The drawing under review shows one solid part. Ordinate dimensions are in mm from its lowest x, y, z. Round coordinates to 2 decimals unless told otherwise and drop trailing zeros. Write each loop counter-clockwise with the first axis right and the second up, starting at its lowest first coordinate (ties: lowest second). Pieces come first, ordered by that corner, then holes. Notation, with made-up numbers: (6, -37) -> (24, -37) arc R26 cw to (24, -14) -> close; hole circle Ø2 at (53.5, -20). An arc over 180 degrees is marked (long way). Use CSV: the item, a comma, the result in double quotes. Start each with the question number.
1) Mouldability with a two-part tool opening along Z and no side actions: class the marked faces 1, 2 and 3 as released by +Z, released by -Z, zero draft, split by the parting line, or undercut.
2) Wall thickness on probe 1 along Z at (x, y) = (1.5, 0.8); probe 2 along Y at (x, z) = (1, 3); probe 3 along Z at (x, y) = (1.05, 0.25): over which ranges is each line inside the solid? List them lowest first. Write a range as [from, to].
3) Take a section at C-C, the plane z = 12.75. Give the boundary of the cut face in (x, y).
4) Take a section at A-A, the plane x = 1. Give the boundary of the cut face in (y, z).
5) For pin 1 Ø1 at (x, z) = (1.5, 14.5) entering from +Y, flat-tipped, find the tip position at first contact; note if it passes through.
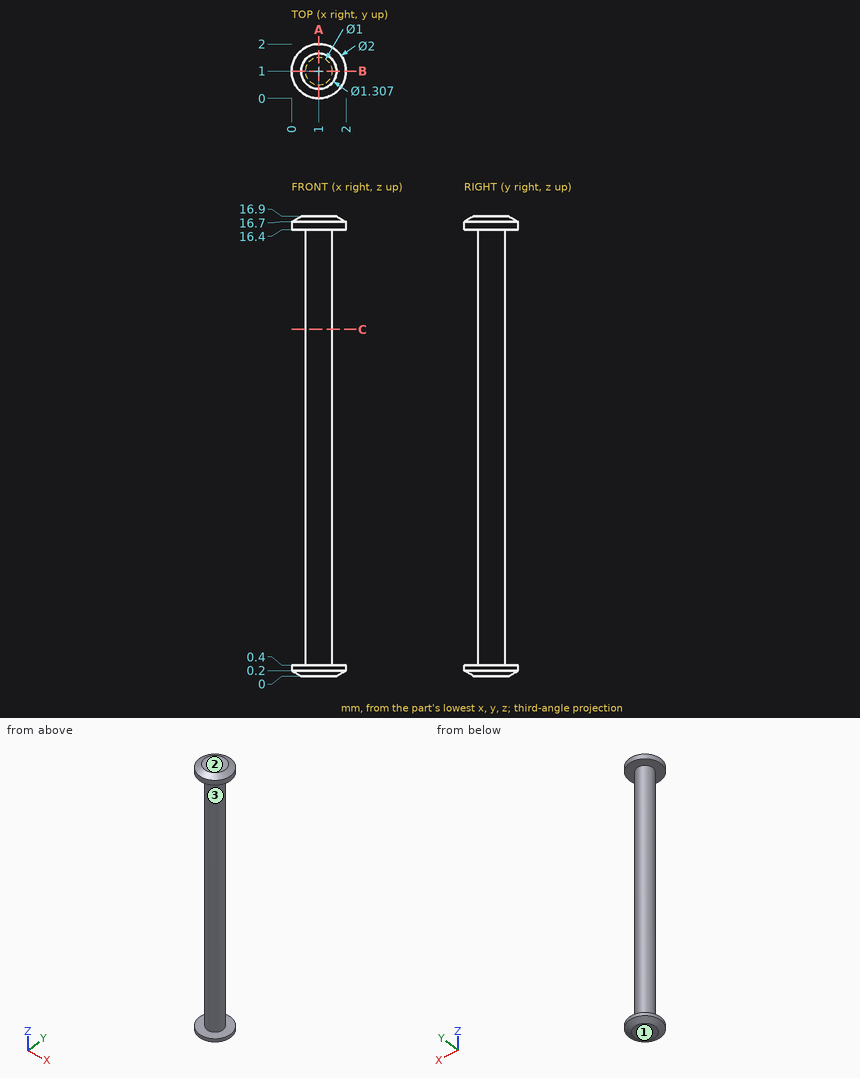
Values found:
1,face 1,"released by -Z"
1,face 2,"released by +Z"
1,face 3,"undercut"
2,probe 1,"[0, 0.4], [16.4, 16.9]"
2,probe 2,"[0.5, 1.5]"
2,probe 3,"[0.06, 0.4], [16.4, 16.84]"
3,outline,"circle Ø1 at (1, 1)"
4,outline,"(0, 0.2) -> (0.35, 0) -> (1.65, 0) -> (2, 0.2) -> (2, 0.4) -> (1.5, 0.4) -> (1.5, 16.4) -> (2, 16.4) -> (2, 16.7) -> (1.65, 16.9) -> (0.35, 16.9) -> (0, 16.7) -> (0, 16.4) -> (0.5, 16.4) -> (0.5, 0.4) -> (0, 0.4) -> close"
5,pin 1,"y = 1.5"
